from build123d import *

# Parameters (mm, degrees)
SKETCH1_R           = 13.5
BOSS_EXTRUDE1_DEPTH = 4.4
SKETCH2_W           = 11.68560188
SKETCH2_H           = 30
SKETCH2_W_2         = 6.209334753
CUT_EXTRUDE2_DEPTH  = 4.4
SKETCH3_R           = 0.6
BOSS_EXTRUDE2_DEPTH = 1.35
SKETCH4_R           = 0.35
BOSS_EXTRUDE3_DEPTH = 0.45
SKETCH5_R           = 0.5
BOSS_EXTRUDE4_DEPTH = 8.25
SKETCH7_R           = 0.085
BOSS_EXTRUDE5_DEPTH = 0.85


with BuildPart() as part:
    # Sketch1 → Boss-Extrude1 (new body)
    with BuildSketch(Plane(origin=(0, 0, 0), x_dir=(1, 0, 0), z_dir=(0, 1, 0))):
        with Locations(Location((0, 0, 0), (0, 0, 270))):
            Circle(SKETCH1_R)
    extrude(amount=BOSS_EXTRUDE1_DEPTH)

    # Sketch2 → Cut-Extrude2 (cut)
    with BuildSketch(Plane(origin=(0, 0, 0), x_dir=(1, 0, 0), z_dir=(0, 1, 0))):
        with Locations((-18.34280094, 0)):
            Rectangle(SKETCH2_W, SKETCH2_H)
        with Locations((15.604667377, 0)):
            Rectangle(SKETCH2_W_2, SKETCH2_H)
    extrude(amount=CUT_EXTRUDE2_DEPTH, mode=Mode.SUBTRACT)

    # Sketch3 → Boss-Extrude2 (add)
    with BuildSketch(Plane(origin=(0, 4.4, 0), x_dir=(1, 0, 0), z_dir=(0, 1, 0))):
        with Locations(Location((0, 0, 0), (0, 0, 270))):
            Circle(SKETCH3_R)
    extrude(amount=BOSS_EXTRUDE2_DEPTH)

    # Sketch4 → Boss-Extrude3 (add)
    with BuildSketch(Plane(origin=(0, 5.75, 0), x_dir=(1, 0, 0), z_dir=(0, 1, 0))):
        with Locations(Location((0, 0, 0), (0, 0, 270))):
            Circle(SKETCH4_R)
    extrude(amount=BOSS_EXTRUDE3_DEPTH)

    # Sketch5 → Boss-Extrude4 (add)
    with BuildSketch(Plane(origin=(12.5, 0, 0), x_dir=(0, 0, -1), z_dir=(1, 0, 0))):
        with Locations((0, 1.55)):
            Circle(SKETCH5_R)
    extrude(amount=BOSS_EXTRUDE4_DEPTH)

    # Sketch7 → Boss-Extrude5 (add)
    with BuildSketch(Plane(origin=(0, 4.4, 0), x_dir=(1, 0, 0), z_dir=(0, 1, 0))):
        with Locations(Location((0, -6.5, 0), (0, 0, 270))):
            Circle(SKETCH7_R)
    extrude(amount=BOSS_EXTRUDE5_DEPTH)


solid = part.part
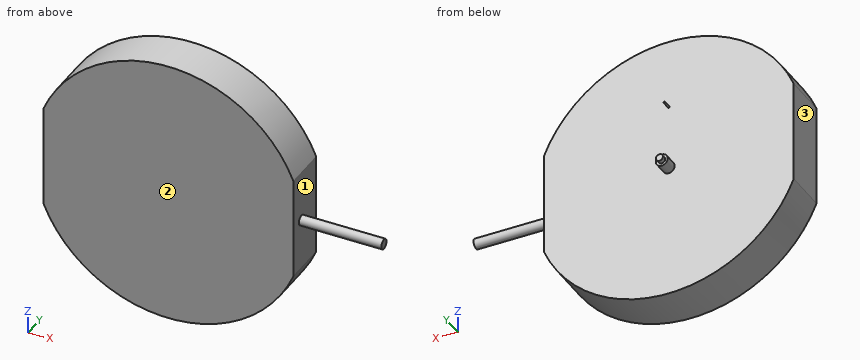
Input: part model. Units: mm. Frame: model coordinates. Face numbers are marked on the shaded views. Round coordinates to 2 decimals unless told otherwise and drop trailing zeros. Write each loop counter-clockwise with the first axis right and the second up, starting at its lowest first coordinate (ties: lowest second). Pieces come first, ordered by that corner, then holes.
1) Ray query, L1, parallel to X at y = 1.25, z = 4.25; L2, parallel to Y at x = 10.5, z = -8; L3, parallel to Z at x = 10, y = 2.5. Return the intervals inside material, ascending.
2) Cut plane B-B (y = 1.55). Return the cut outline in (x, z), then the cut area to 3 significant figures.
3) Draft query along X for the marked faces 1, 2 and 3. Return one class per face: pulls with the +X half, pulls with the -X half, needs draft (parallel to the pull), parting line crosses it, or undercut.
4) Cut plane A-A (z = 0). Return the cut outline in (x, y).
5) Cut plane C-C (x = 16). Return the cut outline in (y, z).
6) Cut plane D-D (z = 4.75). Return the cut outline in (x, y).
7) Contact query for flat-ended pins moving along their axis: P1, Ø3, axis at y = 4.5, z = 10, coming from the -X side; P2, Ø3, axis at x = 6.5, y = 4, coming from the +Z side; P3, Ø2, axis at x = 8, y = 4, coming from the -Z side. Output: stop coordinate, or through.
Geometry says:
1. L1: x = -12.5 to 12.5
1. L2: y = 0 to 4.4
1. L3: z = -9.07 to 9.07
2. outline: (-12.5, -5.1) arc R13.5 ccw to (12.5, -5.1) - (12.5, -0.5) - (20.75, -0.5) - (20.75, 0.5) - (12.5, 0.5) - (12.5, 5.1) arc R13.5 ccw to (-12.5, 5.1) - close
2. area: 567 mm2
3. face 1: pulls with the +X half
3. face 2: needs draft
3. face 3: pulls with the -X half
4. outline: (-12.5, 0) - (12.5, 0) - (12.5, 1.05) - (20.75, 1.05) - (20.75, 2.05) - (12.5, 2.05) - (12.5, 4.4) - (0.6, 4.4) - (0.6, 5.75) - (0.35, 5.75) - (0.35, 6.2) - (-0.35, 6.2) - (-0.35, 5.75) - (-0.6, 5.75) - (-0.6, 4.4) - (-12.5, 4.4) - close
5. outline: circle Ø1 at (1.55, 0)
6. outline: (-12.5, 0) - (12.5, 0) - (12.5, 4.4) - (-12.5, 4.4) - close
7. P1: stops at x = -10.49
7. P2: stops at z = 12.54
7. P3: stops at z = -11.54
